```python
from build123d import *

# Parameters (mm, degrees)
SKETCH1_W           = 1.524
SKETCH1_H           = 1.524
BOSS_EXTRUDE1_DEPTH = 1.524
FILLET1_R           = 2.54


with BuildPart() as part:
    # Sketch1 → Boss-Extrude1 (new body)
    with BuildSketch(Plane.XY):
        Polygon((1.524, -10.497308023), (1.524, -0.972308023), (6.269557814, 4.493617922), (8.055541686, 2.871017969), (7.030741716, 1.743028155), (8.158731531, 0.718228185), (9.183531501, 1.846217999), (10.969515373, 0.223618046), (10.969515373, -3.789821466), (9.188202018, -4.549828763), (9.786265437, -5.951576297), (10.969515373, -5.446736099), (10.969515373, -9.301381954), (9.058811588, -12.009667231), (7.813530127, -11.131117242), (6.934980138, -12.376398702), (8.180261599, -13.254948692), (6.269557814, -15.963233969), align=None)
        with Locations((3.81, -0.762)):
            Rectangle(SKETCH1_W, SKETCH1_H, mode=Mode.SUBTRACT)
    extrude(amount=BOSS_EXTRUDE1_DEPTH)

    # Fillet1
    # the kernel refuses this fillet: 2.54 mm, written as the material it takes off along each edge
    with BuildSketch(Plane(origin=(6.269557814, 4.493617922, -6.477892314), x_dir=(-0.6555947155448552, -0.7551129511203344, 0), z_dir=(0, 0, 1))) as fillet1_piece_1:
        with BuildLine():
            CenterArc((2.591156926, 2.54), FILLET1_R, 182.87981761, 87.12018239)
            Line((0.05436465, 2.412387507), (0.003628804, 2.409835257))
            ThreePointArc((0.003628804, 2.409835257), (-0.023604781, 1.207338273), (-0.050787105, 0.001144519))
            Line((-0.050787105, 0.001144519), (0, -0.0508))
            Line((0, -0.0508), (2.591156926, -0.0508))
            Line((2.591156926, -0.0508), (2.591156926, 0))
        make_face()
    extrude(amount=14.479784629, mode=Mode.SUBTRACT)
    with BuildSketch(Plane(origin=(10.969515373, 0.223618046, -2.81023831), x_dir=(-0.7401507968211615, 0.6724409252603532, 0), z_dir=(0, 0, 1))) as fillet1_piece_2:
        with BuildLine():
            CenterArc((FILLET1_R * 0.442557214214, FILLET1_R), FILLET1_R, 222.255737271, 47.744262729)
            Line((-FILLET1_R * 0.297593582607, FILLET1_R * 0.32755907474), (-FILLET1_R * 0.312396598543, FILLET1_R * 0.314110256234))
            Line((-FILLET1_R * 0.312396598543, FILLET1_R * 0.314110256234), (-FILLET1_R * 0.00885114428429, -FILLET1_R * 0.02))
            Line((-FILLET1_R * 0.00885114428429, -FILLET1_R * 0.02), (FILLET1_R * 0.442557214214, -FILLET1_R * 0.02))
            Line((FILLET1_R * 0.442557214214, -FILLET1_R * 0.02), (FILLET1_R * 0.442557214214, 0))
        make_face()
    extrude(amount=7.144476621, mode=Mode.SUBTRACT)
    with BuildSketch(Plane(origin=(10.969515373, -9.301381954, -2.014527057), x_dir=(0, 1, 0), z_dir=(0, 0, 1))) as fillet1_piece_3:
        with BuildLine():
            CenterArc((FILLET1_R * 0.317248355422, FILLET1_R), FILLET1_R, 234.796910959, 35.203089041)
            Line((-FILLET1_R * 0.259228015403, FILLET1_R * 0.182886180584), (-FILLET1_R * 0.270757542819, FILLET1_R * 0.166543904196))
            Line((-FILLET1_R * 0.270757542819, FILLET1_R * 0.166543904196), (-FILLET1_R * 0.00634496710845, -FILLET1_R * 0.02))
            Line((-FILLET1_R * 0.00634496710845, -FILLET1_R * 0.02), (FILLET1_R * 0.317248355422, -FILLET1_R * 0.02))
            Line((FILLET1_R * 0.317248355422, -FILLET1_R * 0.02), (FILLET1_R * 0.317248355422, 0))
        make_face()
    extrude(amount=5.553054114, mode=Mode.SUBTRACT)
    with BuildSketch(Plane(origin=(6.269557814, -15.963233969, -8.10313634), x_dir=(0.5764763708249786, 0.8171138194159133, 0), z_dir=(0, 0, 1))) as fillet1_piece_4:
        with BuildLine():
            CenterArc((FILLET1_R * 1.27608446293, FILLET1_R), FILLET1_R, 166.167848872, 103.832151128)
            Line((FILLET1_R * 0.305084187293, FILLET1_R * 1.23907836523), (FILLET1_R * 0.28566418178, FILLET1_R * 1.24385993254))
            Line((FILLET1_R * 0.28566418178, FILLET1_R * 1.24385993254), (-FILLET1_R * 0.0255216892585, -FILLET1_R * 0.02))
            Line((-FILLET1_R * 0.0255216892585, -FILLET1_R * 0.02), (FILLET1_R * 1.27608446293, -FILLET1_R * 0.02))
            Line((FILLET1_R * 1.27608446293, -FILLET1_R * 0.02), (FILLET1_R * 1.27608446293, 0))
        make_face()
    extrude(amount=17.730272679, mode=Mode.SUBTRACT)


solid = part.part
```
Geometry: final body of the model. Coordinates: model frame, mm. A direction names the side the tool comes from. Round coordinates to 2 decimals unless told otherwise and drop trailing zeros. Loops run counter-clockwise (first coordinate to the right, second up) from the corner with the lowest first, then second, coordinate; pieces in that order, holes last. Notation, with made-up numbers: (-9, 29) -> (44, 29) arc R24 ccw to (44, 59) -> close; hole circle Ø7 at (63, 33.5). An arc over 180 degrees is marked (long way). Write each question's results on one line, items separated by ' | '.
Item 1: Cut plane C-C on x = 8.5. Return the cut outline in (y, z), and give its area (3 significant figures).
Answers below:
outline: (-11.62, 0) -> (1.09, 0) -> (1.09, 1.52) -> (-11.62, 1.52) -> close | area: 19.4 mm²
Item 2: Pin query (flat end, axial travel): pin 1 Ø0.8 at (x, z) = (4, 0.5) entering from +Y; pin 2 Ø0.8 at (x, z) = (4, 1) entering from -Y; pin 3 Ø0.8 at (y, z) = (-0.5, 0.5) entering from -X. Return the tip coordinate at first contact, or that it passes through.
Answers below:
pin 1: stops at y = 2.34 | pin 2: stops at y = -13.77 | pin 3: stops at x = 1.59
Item 3: Set-up query: faces 5 (the face through (9.79, -10.97, 0.75)), 6 (the face through (8.66, 1.27, 0.75)), 7 (the face through (10.091, -4.165, 0.751)), 8 (the face through (3.048, -1, 1)), 9 (the face through (1.524, -6, 1)). Return all of +Z, -Z, +X, -X, +Y, -Y with unobstructed straight access to the full face (end or side cutting, diameter ignored); none if empty.
Answers below:
face 5: +Z, -Z, +X, -Y | face 6: +Z, -Z, +Y | face 7: +Z, -Z, +X | face 8: +Z, -Z | face 9: +Z, -Z, -X, +Y, -Y
Item 4: Cut plane A-A on z = 1.2. Return the cut outline in (x, y).
Answers below:
outline: (1.52, -10.5) -> (4.14, -13.52) arc R2.54 ccw to (8.14, -13.31) -> (8.18, -13.25) -> (6.93, -12.38) -> (7.81, -11.13) -> (9.06, -12.01) -> (10.5, -9.96) arc R2.54 ccw to (10.97, -8.5) -> (10.97, -5.45) -> (9.79, -5.95) -> (9.19, -4.55) -> (10.97, -3.79) -> (10.97, -0.9) arc R2.54 ccw to (10.14, 0.98) -> (9.18, 1.85) -> (8.16, 0.72) -> (7.03, 1.74) -> (8.06, 2.87) arc R2.54 ccw to (4.57, 2.54) -> (1.52, -0.97) -> close; hole (3.05, -1.52) -> (4.57, -1.52) -> (4.57, 0) -> (3.05, 0) -> close
Item 5: Line query: probe 1 along X at (y, z) = (-1, 0.4); probe 2 along Y at (x, z) = (7.25, 0.7); probe 3 along Y at (x, z) = (4.5, 0.2). Output: solid intervals per line, ascending. Write a range as [from, to].
Answers below:
probe 1: x = [1.52, 3.05], [4.57, 10.97] | probe 2: y = [-14.1, -12.6], [-11.93, 1.54], [1.98, 3.3] | probe 3: y = [-13.85, -1.52], [0, 2.46]
Item 6: Pull-direction query (X, two-part tool) for faces 1 (the face through (3.03, 0.76, 0.75)), 2 (the face through (6, -5, 1.524)), 3 (the face through (4.572, -1, 1)), 4 (the face through (8.445, -11.577, 0.751)); classes: pulls with the +X half, pulls with the -X half, needs draft (parallel to the pull), parting line crosses it, or undercut.
Answers below:
face 1: pulls with the -X half | face 2: needs draft | face 3: undercut | face 4: undercut
Item 7: Cut plane B-B on y = -4. Return the cut outline in (x, z), and give its area (3 significant figures).
Answers below:
outline: (1.52, 0) -> (10.48, 0) -> (10.48, 1.52) -> (1.52, 1.52) -> close | area: 13.6 mm²
